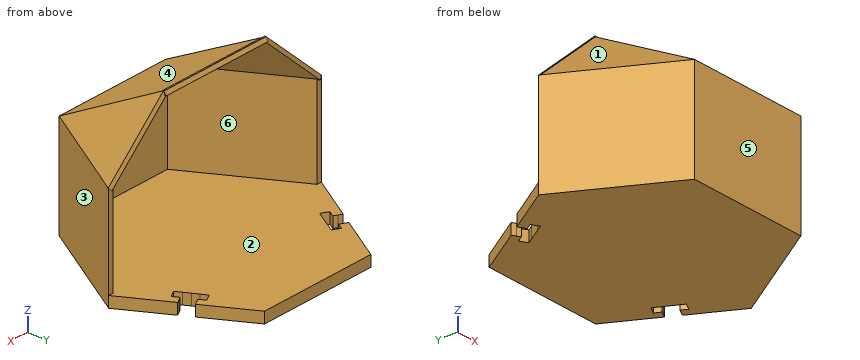
from build123d import *

# Parameters (mm, degrees)
F0_W      = 50
F0_H      = 12.5
F1_DEPTH  = 8
F2_DEPTH  = 75
F4_DEPTH  = 8
F7_DEPTH  = 3
F8_DEPTH  = 1
F11_DEPTH = 3
F14_DEPTH = 3
F15_DEPTH = 8
F16_DEPTH = 25
F17_DEPTH = 8


# Not quite as in the source:
# - a feature names something its author has since deleted; it is built from what else it names


with BuildPart() as f1:
    # F0 (on Top) → F1 (new body)
    with BuildSketch(Plane.XY):
        Polygon((-42.0179491924, 72.7772228311), (-60.5095952989, 40.7487522591), (-57.9695070384, 39.3207329262), (-55.5194165334, 43.6791064608), (-50.2642610162, 40.7248836223), (-52.7144317239, 36.366367418), (-57.615009792, 27.6494680496), (-60.0654171506, 23.2910848888), (-65.3204122546, 26.2455930623), (-62.870004896, 30.6039762231), (-65.5097997054, 32.0881441788), (-84.0358983849, 0), (-42.0179491924, -72.7772228311), (42.0179491924, -72.7772228311), (84.0358983849, 0), (65.5097997054, 32.0881441788), (62.870004896, 30.6039762231), (65.3204122546, 26.2455930623), (60.0654171506, 23.2910848888), (57.615009792, 27.6494680496), (55.164720758, 32.0079177338), (52.7144317239, 36.366367418), (50.2642610162, 40.7248836223), (55.5194165334, 43.6791064608), (57.9695070384, 39.3207329262), (60.5095952989, 40.7487522591), (42.0179491924, 72.7772228311), align=None)
        with Locations((0, 54.5829171234)):
            Rectangle(F0_W, F0_H, mode=Mode.SUBTRACT)
    extrude(amount=F1_DEPTH)

    # F0 (on Top) → F2 (join)
    with BuildSketch(Plane.XY):
        Polygon((43.75, -75.7772228311), (87.5, 0), (84.0358983849, 0), (42.0179491924, -72.7772228311), (-42.0179491924, -72.7772228311), (-84.0358983849, 0), (-87.5, 0), (-43.75, -75.7772228311), align=None)
    extrude(amount=F2_DEPTH)

    # F0 (on Top) → F4 (join)
    with BuildSketch(Plane.XY):
        Polygon((43.75, 75.7772228311), (-43.75, 75.7772228311), (-63.1248363216, 42.2190219338), (-60.5095952989, 40.7487522591), (-42.0179491924, 72.7772228311), (42.0179491924, 72.7772228311), (60.5095952989, 40.7487522591), (63.1248363216, 42.2190219338), align=None)
    extrude(amount=F4_DEPTH)

    # F6 (on face) → F7 (join)
    with BuildSketch(Plane(origin=(0, -50.1312366318, 89.3836679776), x_dir=(1, 0, 0), z_dir=(0, 0.4891706574, -0.872188092))):
        Polygon((43.75, 29.4041920927), (0, 29.4041920927), (-43.75, 29.4041920927), (-42.01795, -57.4775522498), (42.01795, -57.4775522498), align=None)
    extrude(amount=F7_DEPTH)

    # F3 (on Front) → F8 (join)
    with BuildSketch(Plane.XZ):
        Polygon((-42.01795, 114.5), (0, 114.5), (42.01795, 114.5), (84.0359, 75), (87.5, 75), (42.01795, 117.5), (0, 117.5), (-42.01795, 117.5), (-87.5, 75), (-84.0359, 75), align=None)
    extrude(amount=F8_DEPTH)

    # F10 (on face) → F11 (join)
    with BuildSketch(Plane(origin=(-67.6846727043, -39.0777640058, 72.4338274863), x_dir=(0.7723629594, -0.3015876344, 0.5590173143), z_dir=(-0.6351814378, -0.3667221741, 0.6797495039))):
        Polygon((33.2314262259, 55.789645187), (-25.6554603702, 35.6104118215), (30.9888924807, -31.0804218073), align=None)
    extrude(amount=-F11_DEPTH)

    # F13 (on face) → F14 (join)
    with BuildSketch(Plane(origin=(67.6756688636, -39.5950852503, 72.4241918832), x_dir=(0.7733047167, 0.3041472681, -0.556322078), z_dir=(-0.6340345536, 0.3709553614, -0.6785221475))):
        Polygon((-30.939509805, 30.5117392321), (-32.8751652468, -56.3649154418), (25.9400068576, -35.9776056011), align=None)
    extrude(amount=F14_DEPTH)

    # F0 (on Top) → F15 (join)
    with BuildSketch(Plane.XY):
        with Locations((0, 54.5829171234)):
            Rectangle(F0_W, F0_H)
    extrude(amount=F15_DEPTH)

    # F0 (on Top) → F16 (cut)
    with BuildSketch(Plane.XY):
        Polygon((-57.9695070384, 39.3207329262), (-60.5095952989, 40.7487522591), (-65.5097997054, 32.0881441788), (-62.870004896, 30.6039762231), (-57.615009792, 27.6494680496), (-52.7144317239, 36.366367418), align=None)
    extrude(amount=-F16_DEPTH, mode=Mode.SUBTRACT)

    # F0 (on Top) → F17 (join)
    with BuildSketch(Plane.XY):
        Polygon((-65.5097997054, 32.0881441788), (-68.125, 33.5584843966), (-87.5, 0), (-84.0358983849, 0), align=None)
        Polygon((87.5, 0), (68.125, 33.5584843966), (65.5097997054, 32.0881441788), (84.0358983849, 0), align=None)
    extrude(amount=F17_DEPTH)


solid = f1.part
For this review, take the finished solid that the model builds, in its own axes (mm). Face numbers are marked on the shaded views. A direction names the side the tool comes from. Give positions to 0.01 mm unless a question says otherwise; leave off trailing zeros. Loops run counter-clockwise (first coordinate to the right, second up) from the corner with the lowest first, then second, coordinate; pieces in that order, holes last. Notation, with made-up numbers: M 68,-23.5 L 84,-23.5 A18 cw 84,-1.5 Z; hole C 74.25,-3.75 d10. An arc over 180 degrees is marked long. Answer as a JSON object with one key per item and string values. Group by question number.
Q1. Add section A-A on y = -33.5. Give the boundary of the cut face in (x, z), and give its area (3 significant figures).
Q2. Add section B-B on x = -15.5. Give the boundary of the cut face in (y, z), and give its area (3 significant figures).
Q3. For probe 1 along Y at (x, z) = (12.5, 27); probe 2 along Z at (x, y) = (24.5, 47); probe 3 along X at (y, z) = (-28, 83.5), list the stretches that pass through material, from the lowest coordinate up. Write a range as [from, to].
Q4. Mouldability with a two-part tool opening along Z and no side actions: class the marked faces 1, 2 and 3 as +Z half, -Z half, draft (parallel to the pull), parting line (faces both ways), or undercut.
Q5. Add section D-D on y = -58. Give the boundary of the cut face in (x, z).
Q6. Add section C-C on z = 63. Give the boundary of the cut face in (x, y), and give its area (3 significant figures).
Q7. Tool access review of the marked faces 4, 5 and 6: name each direction out of +Z, -Z, +X, -X, +Y, -Y from which nothing blocks a thin tool from reaching the whole face with its end or side.
Q8. Insertion check: P1, Ø1, axis at x = -47, z = 45.5, coming from the -Y side; P2, Ø1.7, axis at x = -85.5, z = 42, coming from the +Y side; P3, Ø1, axis at x = 54.5, z = 103, coming from the +Y side. Each pin has a flat end and moves straight along its axis. Give the tip position at first contact, or say it passes through.
Checked values:
{
 "1": {"outline": "M -68.16,0 L 68.16,0 L 68.16,75 L 68.33,75.14 L 42.91,98.9 L 42.78,98.71 L -42.78,98.71 L -68.16,75 Z; hole M -64.69,8 L 64.69,8 L 64.69,74.12 L 42.06,95.27 L -41.74,95.27 L -64.69,73.82 Z", "area": "2,060 mm²"},
 "2": {"outline": "M -75.78,0 L 75.78,0 L 75.78,8 L -72.78,8 L -72.78,73.24 L 1.47,114.88 L 0,117.5 L -1,117.5 L -1,116.94 L -75.78,75 Z", "area": "1,670 mm²"},
 "3": {"probe 1": "[-75.78, -72.78]", "probe 2": "[0, 8]", "probe 3": "[-62.24, -57.51], [57.88, 62.61]"},
 "4": {"face 1": "+Z half", "face 2": "undercut", "face 3": "draft"},
 "5": {"outline": "M -54.01,0 L 54.01,0 L 54.01,75 L 54.09,75.06 L 43.4,85.05 L 43.34,84.97 L -43.34,84.97 L -54.01,75 Z; hole M -50.55,8 L 50.55,8 L 50.55,73.94 L 42.43,81.53 L -42.3,81.53 L -50.55,73.82 Z"},
 "6": {"outline": "M -87.5,0 L -43.75,-75.78 L 43.75,-75.78 L 87.5,0 L 84.04,0 L 42.02,-72.78 L -42.02,-72.78 L -84.04,0 Z", "area": "772 mm²"},
 "7": {"face 4": "+Z, -X, -Y", "face 5": "+Z, -Z, +X, -X, -Y", "face 6": "+Y"},
 "8": {"P1": "y = -71.01", "P2": "y = 0", "P3": "y = 0.98"}
}
